from build123d import *

# Parameters (mm, degrees)
F1_DEPTH = 224
F3_D     = 8
F5_D     = 8


with BuildPart() as f1:
    # F0 (on Right) → F1 (new body)
    with BuildSketch(Plane.YZ):
        Polygon((0, 30), (0, 0), (30, 0), (30, 3), (3, 3), (3, 30), align=None)
    extrude(amount=F1_DEPTH)

    # F3 (through all)
    with Locations(Plane(origin=(0, 0, 0), x_dir=(1, 0, 0), z_dir=(0, 0, -1))):
        with Locations((15, -15), (100, -15.3021634132), (209, -15.3983095661)):
            Hole(F3_D / 2)

    # F5 (through all)
    with Locations(Plane.XZ):
        with Locations((30, 15), (120, 15), (195, 15)):
            Hole(F5_D / 2)


solid = f1.part
Source: CAD feature listing. Evaluate the final solid. Frame: model axes, mm. A direction names the side the tool comes from. Give positions to 0.01 mm unless a question says otherwise; leave off trailing zeros. Write each loop counter-clockwise with the first axis right and the second up, starting at its lowest first coordinate (ties: lowest second). Pieces come first, ordered by that corner, then holes. Notation, with made-up numbers: (35.5, 9) -> (40.5, 9) arc R21 ccw to (40.5, 16) -> close; hole circle Ø6 at (-25, -39.75). An arc over 180 degrees is marked (long way). Return JSON: item names as keys, results as strings. Group by question number.
1. Section A-A, the plane x = 30. Output: boundary loops of the cut face in (y, z), then the cut area to 3 significant figures.
2. Material intervals for line 1 (Y direction, x = 15, z = 2.3); line 2 (Y direction, x = 209, z = 2.05), sorted ascending. Write a range as from..to.
3. Pin query (flat end, axial travel): pin 1 Ø3 at (x, z) = (126, 9.5) entering from +Y; pin 2 Ø6.5 at (x, y) = (15, 15) entering from +Z; pin 3 Ø10 at (x, y) = (192, 17) entering from +Z. Return the tip coordinate at first contact, or that it passes through.
4. Section C-C, the plane x = 174. Output: boundary loops of the cut face in (y, z), then the cut area to 3 significant figures.
5. Section D-D, the plane z = 26.75. Output: boundary loops of the cut face in (x, y).
6. Mould query, pull axis Y, two halves, no side actions, for faces 1 (the face through (110, 3, 16)), 2 (the face through (110, 15, 0)), 3 (the face through (209.867, 19.303, 1.521)), 4 (the face through (110, 0, 15)). Classes: +Y half, -Y half, draft (parallel to the pull), parting line (faces both ways), or undercut.
7. Access query for faces 5 (the face through (110, 17, 3)), 6 (the face through (19, 15, 2)). Directions: +Z, -Z, +X, -X, +Y, -Y. A direction counts if a zero-diameter tool reaches every point of the face in a straight line with its end or side. Return the directions, or none.
8. Section B-B, the plane z = 13. Output: boundary loops of the cut face in (x, y).
Determined:
{
 "1": {"outline": "(0, 0) -> (30, 0) -> (30, 3) -> (3, 3) -> (3, 11) -> (0, 11) -> close; (0, 19) -> (3, 19) -> (3, 30) -> (0, 30) -> close", "area": "147 mm2"},
 "2": {"line 1": "y = 0..11, 19..30", "line 2": "y = 0..11.4, 19.4..30"},
 "3": {"pin 1": "stops at y = 3", "pin 2": "passes through", "pin 3": "stops at z = 3"},
 "4": {"outline": "(0, 0) -> (30, 0) -> (30, 3) -> (3, 3) -> (3, 30) -> (0, 30) -> close", "area": "171 mm2"},
 "5": {"outline": "(0, 0) -> (224, 0) -> (224, 3) -> (0, 3) -> close"},
 "6": {"face 1": "+Y half", "face 2": "draft", "face 3": "undercut", "face 4": "-Y half"},
 "7": {"face 5": "+Z, +X, -X, +Y", "face 6": "+Z, -Z"},
 "8": {"outline": "(0, 0) -> (26.54, 0) -> (26.54, 3) -> (0, 3) -> close; (33.46, 0) -> (116.54, 0) -> (116.54, 3) -> (33.46, 3) -> close; (123.46, 0) -> (191.54, 0) -> (191.54, 3) -> (123.46, 3) -> close; (198.46, 0) -> (224, 0) -> (224, 3) -> (198.46, 3) -> close"}
}
